Input: part model. Units: mm. Frame: model coordinates. Face numbers are marked on the shaded views. A direction names the side the tool comes from. Coordinates: 2 decimals unless noted, no trailing zeros. Order: outer loops, then holes, each group sorted by start corner. A loop starts at its lowest first (then second) coordinate and runs counter-clockwise, first axis right, second up. Notation, with made-up numbers: M 22,51.25 L 31,51.25 A33 cw 31,84.25 Z; hole C 72.25,-28 d3. An arc over 180 degrees is marked long. Answer in a Markdown table with one row per item.
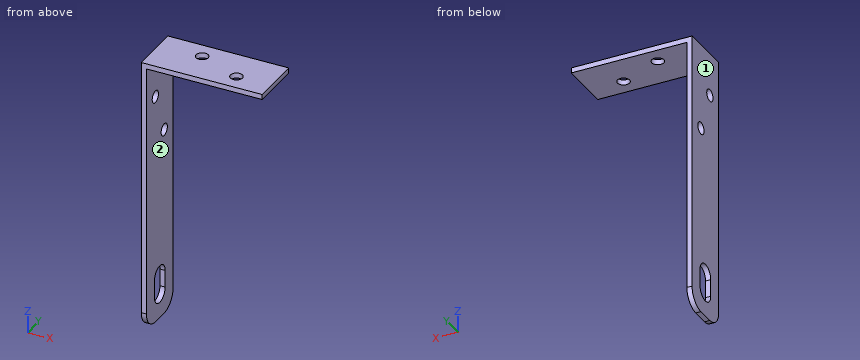
from build123d import *

# Parameters (mm, degrees)
EXTRUDE_1_DEPTH     = 30
SKETCH_2_R          = 3.5
CUT_EXTRUDE_1_DEPTH = 71
SKETCH_3_R          = 3.5
CUT_EXTRUDE_2_DEPTH = 161
CUT_EXTRUDE_3_DEPTH = 71


with BuildPart() as part:
    # Эскиз1 → Вытянуть-Тонкостенный1 (new body)
    with BuildSketch(Plane(origin=(0, 0, 0), x_dir=(1, 0, 0), z_dir=(0, 1, 0))):
        Polygon((0, 160), (0, 120), (0, 0), (70, 0), (70, 3), (3, 3), (3, 120), (3, 160), align=None)
    extrude(amount=EXTRUDE_1_DEPTH)

    # Эскиз2 → Вырез-Вытянуть1 (cut, through all)
    with BuildSketch(Plane.ZY):
        with Locations((-50, 20)):
            Circle(SKETCH_2_R)
        with Locations((-25, 10)):
            Circle(SKETCH_2_R)
    extrude(amount=-CUT_EXTRUDE_1_DEPTH, mode=Mode.SUBTRACT)

    # Эскиз3 → Вырез-Вытянуть2 (cut, through all)
    with BuildSketch(Plane.XY):
        with Locations((25, 20)):
            Circle(SKETCH_3_R)
        with Locations((50, 10)):
            Circle(SKETCH_3_R)
    extrude(amount=-CUT_EXTRUDE_2_DEPTH, mode=Mode.SUBTRACT)

    # Эскиз4 → Вырез-Вытянуть3 (cut, through all)
    with BuildSketch(Plane.ZY):
        with BuildLine():
            Line((-145, 21), (-135, 21))
            ThreePointArc((-135, 21), (-129, 15), (-135, 9))
            Line((-135, 9), (-145, 9))
            ThreePointArc((-145, 9), (-151, 15), (-145, 21))
        make_face()
        with BuildLine():
            Line((-160, 20), (-160, 30))
            Line((-160, 30), (-150, 30))
            ThreePointArc((-150, 30), (-157.071067812, 27.071067812), (-160, 20))
        make_face()
        with BuildLine():
            Line((-160, 10), (-160, 0))
            Line((-160, 0), (-150, 0))
            ThreePointArc((-150, 0), (-157.071067812, 2.928932188), (-160, 10))
        make_face()
    extrude(amount=-CUT_EXTRUDE_3_DEPTH, mode=Mode.SUBTRACT)


solid = part.part
1) Cut plane C-C, the plane x = 40.5. Output: boundary loops of the cut face in (y, z).
Resolved:
| item | result |
|---|---|
| outline | M 0,-3 L 30,-3 L 30,0 L 0,0 Z |
2) Cut plane A-A, the plane x = 50. Output: boundary loops of the cut face in (y, z), and give its area (3 significant figures).
Resolved:
| item | result |
|---|---|
| outline | M 0,-3 L 6.5,-3 L 6.5,0 L 0,0 Z; M 13.5,-3 L 30,-3 L 30,0 L 13.5,0 Z |
| area | 69.0 mm2 |
3) Cut plane B-B, the plane z = -25. Output: boundary loops of the cut face in (x, y).
Resolved:
| item | result |
|---|---|
| outline | M 0,0 L 3,0 L 3,6.5 L 0,6.5 Z; M 0,13.5 L 3,13.5 L 3,30 L 0,30 Z |
4) Cut plane D-D, the plane y = 2.75. Output: boundary loops of the cut face in (x, z), and give its area (3 significant figures).
Resolved:
| item | result |
|---|---|
| outline | M 0,-156.89 L 3,-156.89 L 3,-3 L 70,-3 L 70,0 L 0,0 Z |
| area | 672 mm2 |
5) Reachability of the marked faces 1 and 2 from +Z, -Z, +X, -X, +Y, -Y: full face, straight path, thin tool, end or side. Return the list, or none.
Resolved:
| item | result |
|---|---|
| face 1 | +Z, -Z, -X, +Y, -Y |
| face 2 | -Z, +X, +Y, -Y |
6) Contact query for flat-ended pins moving along their axis: pin 1 (15 mm diameter, centred on y = 21, z = -92.5, fed in from +X); pin 2 (1.5 mm diameter, centred on x = 52, y = 6, fed in from -Z); pin 3 (4 mm diameter, centred on y = 10, z = -25, fed in from +X). Output: stop coordinate, or through.
Resolved:
| item | result |
|---|---|
| pin 1 | stops at x = 3 |
| pin 2 | stops at z = -3 |
| pin 3 | passes through |
7) Material intervals for probe 1 along Y at (x, z) = (1.9, -50); probe 2 along Y at (x, z) = (50, -1); probe 3 along X at (y, z) = (16.5, -74), sorted ascending.
Resolved:
| item | result |
|---|---|
| probe 1 | y = 0 to 16.5, 23.5 to 30 |
| probe 2 | y = 0 to 6.5, 13.5 to 30 |
| probe 3 | x = 0 to 3 |
